```python
from build123d import *

# Parameters (mm, degrees)
SKETCH_1_W          = 9
SKETCH_1_H          = 6.5
EXTRUDE_1_DEPTH     = 608
SKETCH_2_R          = 1.75
CUT_EXTRUDE_1_DEPTH = 7.5
SKETCH_3_R          = 3.25
CUT_EXTRUDE_2_DEPTH = 3.5
CUT_EXTRUDE_3_DEPTH = 609
SKETCH_5_R          = 3.25
CUT_EXTRUDE_4_DEPTH = 3.5
SKETCH_6_R          = 1.75
CUT_EXTRUDE_5_DEPTH = 4
SKETCH_7_W          = 9
SKETCH_7_H          = 3
CUT_EXTRUDE_6_DEPTH = 7.5


with BuildPart() as part:
    # 草图1 → 凸台-拉伸1 (new body)
    with BuildSketch(Plane.XY):
        Rectangle(SKETCH_1_W, SKETCH_1_H)
    extrude(amount=EXTRUDE_1_DEPTH)

    # 草图2 → 切除-拉伸1 (cut, through all)
    with BuildSketch(Plane(origin=(0, 3.25, 0), x_dir=(1, 0, 0), z_dir=(0, 1, 0))):
        with Locations((0, -7.5)):
            Circle(SKETCH_2_R)
        with Locations((0, -27.5)):
            Circle(SKETCH_2_R)
        with Locations((0, -47.5)):
            Circle(SKETCH_2_R)
        with Locations((0, -67.5)):
            Circle(SKETCH_2_R)
        with Locations((0, -87.5)):
            Circle(SKETCH_2_R)
        with Locations((0, -107.5)):
            Circle(SKETCH_2_R)
        with Locations((0, -127.5)):
            Circle(SKETCH_2_R)
        with Locations((0, -147.5)):
            Circle(SKETCH_2_R)
        with Locations((0, -167.5)):
            Circle(SKETCH_2_R)
        with Locations((0, -187.5)):
            Circle(SKETCH_2_R)
        with Locations((0, -207.5)):
            Circle(SKETCH_2_R)
        with Locations((0, -227.5)):
            Circle(SKETCH_2_R)
        with Locations((0, -247.5)):
            Circle(SKETCH_2_R)
        with Locations((0, -267.5)):
            Circle(SKETCH_2_R)
        with Locations((0, -287.5)):
            Circle(SKETCH_2_R)
        with Locations((0, -307.5)):
            Circle(SKETCH_2_R)
        with Locations((0, -327.5)):
            Circle(SKETCH_2_R)
        with Locations((0, -347.5)):
            Circle(SKETCH_2_R)
        with Locations((0, -367.5)):
            Circle(SKETCH_2_R)
        with Locations((0, -387.5)):
            Circle(SKETCH_2_R)
    extrude(amount=-CUT_EXTRUDE_1_DEPTH, mode=Mode.SUBTRACT)

    # 草图3 → 切除-拉伸2 (cut)
    with BuildSketch(Plane(origin=(0, 3.25, 0), x_dir=(1, 0, 0), z_dir=(0, 1, 0))):
        with Locations((0, -7.5)):
            Circle(SKETCH_3_R)
        with Locations((0, -27.5)):
            Circle(SKETCH_3_R)
        with Locations((0, -47.5)):
            Circle(SKETCH_3_R)
        with Locations((0, -67.5)):
            Circle(SKETCH_3_R)
        with Locations((0, -87.5)):
            Circle(SKETCH_3_R)
        with Locations((0, -107.5)):
            Circle(SKETCH_3_R)
        with Locations((0, -127.5)):
            Circle(SKETCH_3_R)
        with Locations((0, -147.5)):
            Circle(SKETCH_3_R)
        with Locations((0, -167.5)):
            Circle(SKETCH_3_R)
        with Locations((0, -187.5)):
            Circle(SKETCH_3_R)
        with Locations((0, -207.5)):
            Circle(SKETCH_3_R)
        with Locations((0, -227.5)):
            Circle(SKETCH_3_R)
        with Locations((0, -247.5)):
            Circle(SKETCH_3_R)
        with Locations((0, -267.5)):
            Circle(SKETCH_3_R)
        with Locations((0, -287.5)):
            Circle(SKETCH_3_R)
        with Locations((0, -307.5)):
            Circle(SKETCH_3_R)
        with Locations((0, -327.5)):
            Circle(SKETCH_3_R)
        with Locations((0, -347.5)):
            Circle(SKETCH_3_R)
        with Locations((0, -367.5)):
            Circle(SKETCH_3_R)
        with Locations((0, -387.5)):
            Circle(SKETCH_3_R)
    extrude(amount=-CUT_EXTRUDE_2_DEPTH, mode=Mode.SUBTRACT)

    # 草图4 → 切除-拉伸3 (cut, through all)
    with BuildSketch(Plane(origin=(0, 0, 0), x_dir=(-1, 0, 0), z_dir=(0, 0, -1))):
        Polygon((4.5, -0.25), (3.5, -0.45), (3.5, -1.05), (4.5, -1.25), align=None)
        Polygon((-4.5, -0.25), (-3.5, -0.45), (-3.5, -1.05), (-4.5, -1.25), align=None)
    extrude(amount=-CUT_EXTRUDE_3_DEPTH, mode=Mode.SUBTRACT)

    # 草图5 → 切除-拉伸4 (cut)
    with BuildSketch(Plane(origin=(0, 3.25, 0), x_dir=(1, 0, 0), z_dir=(0, 1, 0))):
        with Locations((0, -407.5)):
            Circle(SKETCH_5_R)
        with Locations((0, -427.5)):
            Circle(SKETCH_5_R)
        with Locations((0, -447.5)):
            Circle(SKETCH_5_R)
        with Locations((0, -467.5)):
            Circle(SKETCH_5_R)
        with Locations((0, -487.5)):
            Circle(SKETCH_5_R)
        with Locations((0, -507.5)):
            Circle(SKETCH_5_R)
        with Locations((0, -527.5)):
            Circle(SKETCH_5_R)
        with Locations((0, -547.5)):
            Circle(SKETCH_5_R)
        with Locations((0, -567.5)):
            Circle(SKETCH_5_R)
        with Locations((0, -587.5)):
            Circle(SKETCH_5_R)
    extrude(amount=-CUT_EXTRUDE_4_DEPTH, mode=Mode.SUBTRACT)

    # 草图6 → 切除-拉伸5 (cut, through all)
    with BuildSketch(Plane(origin=(0, -0.25, 0), x_dir=(1, 0, 0), z_dir=(0, 1, 0))):
        with Locations((0, -407.5)):
            Circle(SKETCH_6_R)
        with Locations((0, -427.5)):
            Circle(SKETCH_6_R)
        with Locations((0, -447.5)):
            Circle(SKETCH_6_R)
        with Locations((0, -467.5)):
            Circle(SKETCH_6_R)
        with Locations((0, -487.5)):
            Circle(SKETCH_6_R)
        with Locations((0, -507.5)):
            Circle(SKETCH_6_R)
        with Locations((0, -527.5)):
            Circle(SKETCH_6_R)
        with Locations((0, -547.5)):
            Circle(SKETCH_6_R)
        with Locations((0, -567.5)):
            Circle(SKETCH_6_R)
        with Locations((0, -587.5)):
            Circle(SKETCH_6_R)
    extrude(amount=-CUT_EXTRUDE_5_DEPTH, mode=Mode.SUBTRACT)

    # 草图7 → 切除-拉伸6 (cut, through all)
    with BuildSketch(Plane(origin=(0, 3.25, 0), x_dir=(1, 0, 0), z_dir=(0, 1, 0))):
        with Locations((0, -606.5)):
            Rectangle(SKETCH_7_W, SKETCH_7_H)
    extrude(amount=-CUT_EXTRUDE_6_DEPTH, mode=Mode.SUBTRACT)


solid = part.part
```
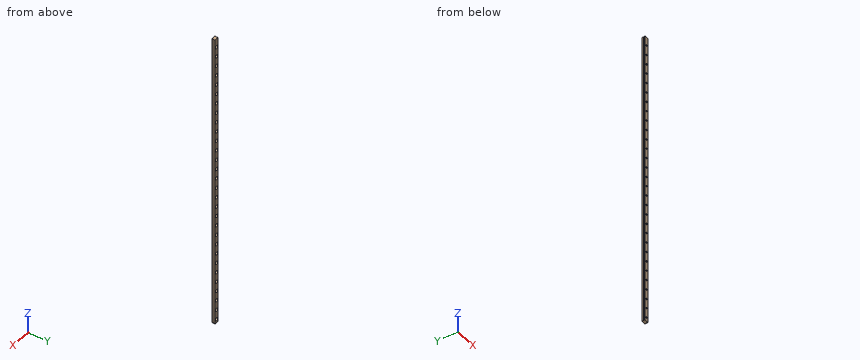
Part model, mm, in its own coordinate system. Round coordinates to 2 decimals unless told otherwise and drop trailing zeros. Write each loop counter-clockwise with the first axis right and the second up, starting at its lowest first coordinate (ties: lowest second). Pieces come first, ordered by that corner, then holes.
Item 1: Cut at A-A, the plane y = 1.5. Count the separate pieces of the cut face and the enclosed holes in it, plus the area to 3 significant figures.
Results:
separate pieces: 1
enclosed holes: 30
area: 4,450 mm2
Item 2: Probe L1, parallel to X at y = -2.35, z = 387.5; L2, parallel to X at y = 1.5, z = 268; L3, parallel to X at y = -1, z = 564. List the from-to ranges inside material, lowest first.
Results:
L1: x = -4.5 to -1.75, 1.75 to 4.5
L2: x = -4.5 to -3.21, 3.21 to 4.5
L3: x = -3.5 to 3.5
Item 3: Drop a flat-ended pin along its axis: pin 1 Ø4 at (x, z) = (0, 507.5) entering from +Y. Give the stop position or say it passes through.
Results:
pin 1: stops at y = -0.25
Item 4: Cut at B-B, the plane z = 217.5. Give the cut face in (x, y).
Results:
outline: (-4.5, -3.25) - (4.5, -3.25) - (4.5, -1.25) - (3.5, -1.05) - (3.5, -0.45) - (4.5, -0.25) - (4.5, 3.25) - (-4.5, 3.25) - (-4.5, -0.25) - (-3.5, -0.45) - (-3.5, -1.05) - (-4.5, -1.25) - close
